For this review, take the finished solid that the model builds, in its own axes (mm). A direction names the side the tool comes from. Round coordinates to 2 decimals unless told otherwise and drop trailing zeros. Order: outer loops, then holes, each group sorted by start corner. A loop starts at its lowest first (then second) coordinate and runs counter-clockwise, first axis right, second up. Notation, with made-up numbers: M -13,-12 L -4,-12 A20 cw -4,5 Z; hole C -21,30 d6. An arc over 180 degrees is marked long. Put each result on its own line as item: value.
from build123d import *

# Parameters (mm, degrees)
SKETCH1_W           = 55.88
SKETCH1_H           = 53.34
BOSS_EXTRUDE1_DEPTH = 104.14
SKETCH2_R           = 8.89
CUT_EXTRUDE1_DEPTH  = 112.072373253
SKETCH3_R           = 20.32
CUT_EXTRUDE2_DEPTH  = 12.7


with BuildPart() as part:
    # Sketch1 → Boss-Extrude1 (new body)
    with BuildSketch(Plane(origin=(0, 0, 0), x_dir=(0, 0, -1), z_dir=(1, 0, 0))):
        Rectangle(SKETCH1_W, SKETCH1_H)
    extrude(amount=BOSS_EXTRUDE1_DEPTH)

    # Sketch2 → Cut-Extrude1 (cut, through all)
    with BuildSketch(Plane(origin=(104.14, 0, 0), x_dir=(0, 0, -1), z_dir=(1, 0, 0))):
        Circle(SKETCH2_R)
    extrude(amount=-CUT_EXTRUDE1_DEPTH, mode=Mode.SUBTRACT)

    # Sketch3 → Cut-Extrude2 (cut)
    with BuildSketch(Plane(origin=(0, 26.67, 0), x_dir=(1, 0, 0), z_dir=(0, 1, 0))):
        with Locations(Location((52.07, 0, 0), (0, 0, 270))):
            Circle(SKETCH3_R)
    extrude(amount=-CUT_EXTRUDE2_DEPTH, mode=Mode.SUBTRACT)


solid = part.part
(1) To check wall thickness, follow L1, parallel to Z at x = 52, y = 20; L2, parallel to Y at x = 68, z = 0; L3, parallel to X at y = 19.25, z = 0. State the ranges of each line that lie inside material, in increasing order.
A:
L1: z = -27.94 to -20.32, 20.32 to 27.94
L2: y = -26.67 to -8.89, 8.89 to 13.97
L3: x = 0 to 31.75, 72.39 to 104.14
(2) Add section B-B on z = 0. Give the boundary of the cut face in (x, y).
A:
outline: M 0,-26.67 L 104.14,-26.67 L 104.14,-8.89 L 0,-8.89 Z; M 0,8.89 L 104.14,8.89 L 104.14,26.67 L 72.39,26.67 L 72.39,13.97 L 31.75,13.97 L 31.75,26.67 L 0,26.67 Z
(3) For faces 1 (the face through (51, 0, -27.94)), 2 (the face through (72.217, 20.409, -2.645)), list the 3-axis set-ups (+Z, -Z, +X, -X, +Y, -Y) from which the entire face can be reached by the end or side of a thin tool; tool diameter is ignored.
A:
face 1: -Z, +X, -X, +Y, -Y
face 2: +Y
(4) Add section C-C on x = 52.07. Give the boundary of the cut face in (y, z), then the cut area to 3 significant figures.
A:
outline: M -26.67,-27.94 L 26.67,-27.94 L 26.67,-20.32 L 13.97,-20.32 L 13.97,20.32 L 26.67,20.32 L 26.67,27.94 L -26.67,27.94 Z; hole C 0,0 d17.78
area: 2,220 mm2
(5) Add section A-A on y = 0. Give the boundary of the cut face in (x, z).
A:
outline: M 0,-27.94 L 104.14,-27.94 L 104.14,-8.89 L 0,-8.89 Z; M 0,8.89 L 104.14,8.89 L 104.14,27.94 L 0,27.94 Z
(6) Insertion check: pin 1 Ø6 at (x, z) = (55, -17) entering from +Y. The pin has a flat end and moves straight along its axis. Give the tip position at first contact, or say it passes through.
A:
pin 1: stops at y = 13.97
(7) Add section D-D on y = 16. Give the boundary of the cut face in (x, z).
A:
outline: M 0,-27.94 L 104.14,-27.94 L 104.14,27.94 L 0,27.94 Z; hole C 52.07,0 d40.64
(8) Draft analysis for pull direction Y (two halves, no side actions). For faces 3 (the face through (52.8, -8.68, 1.93)), 4 (the face through (0, 6, 7)), 5 (the face through (52, 13.97, 0)), state which applies: released by +Y, released by -Y, zero draft, split by the parting line, or undercut.
A:
face 3: undercut
face 4: zero draft
face 5: released by +Y
